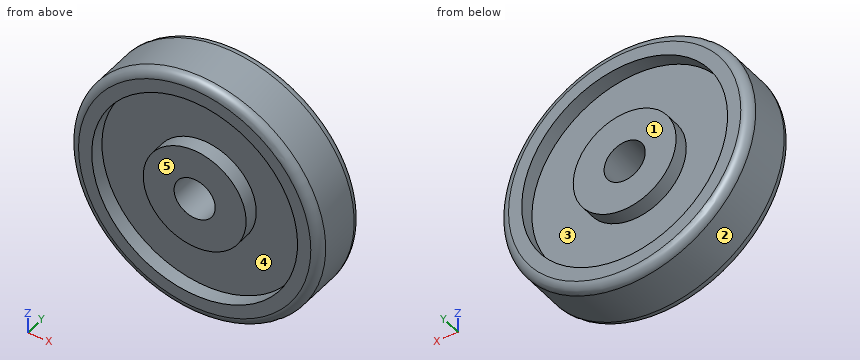
```python
from build123d import *

# Parameters (mm, degrees)
SKETCH_1_R          = 42.5
SKETCH_1_R_2        = 7
EXTRUDE_1_DEPTH     = 20
SKETCH_2_R          = 35
SKETCH_2_R_2        = 17.5
CUT_EXTRUDE_1_DEPTH = 5
CUT_EXTRUDE_START   = -5
SKETCH_3_R          = 35
SKETCH_3_R_2        = 17.5
CUT_EXTRUDE_2_DEPTH = 5
FILLET_1_R          = 3


with BuildPart() as part:
    # 草图1 → 凸台-拉伸1 (new body)
    with BuildSketch(Plane(origin=(0, 0, 0), x_dir=(1, 0, 0), z_dir=(0, 1, 0))):
        with Locations(Location((0, 0, 0), (0, 0, 270))):
            Circle(SKETCH_1_R)
        with Locations(Location((0, 0, 0), (0, 0, 270))):
            Circle(SKETCH_1_R_2, mode=Mode.SUBTRACT)
    extrude(amount=EXTRUDE_1_DEPTH)

    # 草图2 → 切除-拉伸1 (cut)
    with BuildSketch(Plane(origin=(0, 20, 0), x_dir=(1, 0, 0), z_dir=(0, 1, 0))):
        with Locations(Location((0, 0, 0), (0, 0, 270))):
            Circle(SKETCH_2_R)
        with Locations(Location((0, 0, 0), (0, 0, 270))):
            Circle(SKETCH_2_R_2, mode=Mode.SUBTRACT)
    extrude(amount=-CUT_EXTRUDE_1_DEPTH, mode=Mode.SUBTRACT)

    # 草图3 → 切除-拉伸2 (cut)
    with BuildSketch(Plane.XZ.offset(CUT_EXTRUDE_START)):
        with Locations(Location((0, 0, 0), (0, 0, 90))):
            Circle(SKETCH_3_R)
        with Locations(Location((0, 0, 0), (0, 0, 90))):
            Circle(SKETCH_3_R_2, mode=Mode.SUBTRACT)
    extrude(amount=CUT_EXTRUDE_2_DEPTH, mode=Mode.SUBTRACT)

    # 圆角1
    fillet_1_edges = [part.edges().sort_by_distance(p)[0] for p in [
        (0, 0, -42.5),
        (0, 20, -42.5),
    ]]
    fillet(fillet_1_edges, radius=FILLET_1_R)


solid = part.part
```
Could you check a few things on this model? Use its own coordinates, in mm. Face numbers are marked on the shaded views. A direction names the side the tool comes from. Give positions to 0.01 mm unless a question says otherwise; leave off trailing zeros. Order: outer loops, then holes, each group sorted by start corner. A loop starts at its lowest first (then second) coordinate and runs counter-clockwise, first axis right, second up.
Q1. If I drill on line 1 along X through (y, z) = (16.6, 0); line 2 along X through (y, z) = (4.75, 9.5); line 3 along Z through (x, y) = (-6, 1.25), over which ranges is the centre line in solid material (lowest first)?
Q2. Suppose I cut it at B-B, the plane z = 0. Write out the boundary of the cut face in (x, y), and give its area (3 significant figures).
Q3. For the marked faces 4 and 5, which set-ups out of +Z, -Z, +X, -X, +Y, -Y let a thin tool reach every point of the face, with its end or its side?
Q4. I'm going to push flat-ended pins straight in: P1, Ø3, axis at x = -24, z = -18.5, coming from the -Y side; P2, Ø12, axis at y = 15.5, z = 18.5, coming from the -X side; P3, Ø1.5, axis at x = 13.5, y = 16, coming from the +Z side. Where does each tip first touch, or does it pass through?
Q5. We'd pull the mould along X, two halves only. Please class the marked faces 1, 2 and 3: +X half, -X half, draft (parallel to the pull), parting line (faces both ways), or undercut.
Q6. Suppose I cut it at A-A, the plane x = 0. Write out the boundary of the cut face in (y, z), and give its area (3 significant figures).
Q7. Suppose I cut it at C-C, the plane y = 18. Write out the boundary of the cut face in (x, z), and give its area (3 significant figures).
Q8. Suppose I cut it at D-D, the plane y = 12. Write out the boundary of the cut face in (x, z), and give its area (3 significant figures).
Solution:
1. line 1: x = -42.5 to -35, -17.5 to -7, 7 to 17.5, 35 to 42.5
1. line 2: x = -41.42 to -33.69, -14.7 to 14.7, 33.69 to 41.42
1. line 3: z = -41.51 to -34.48, -16.44 to -3.61, 3.61 to 16.44, 34.48 to 41.51
2. outline: (-42.5, 3) arc R3 ccw to (-39.5, 0) - (-35, 0) - (-35, 5) - (-17.5, 5) - (-17.5, 0) - (-7, 0) - (-7, 20) - (-17.5, 20) - (-17.5, 15) - (-35, 15) - (-35, 20) - (-39.5, 20) arc R3 ccw to (-42.5, 17) - close; (7, 0) - (17.5, 0) - (17.5, 5) - (35, 5) - (35, 0) - (39.5, 0) arc R3 ccw to (42.5, 3) - (42.5, 17) arc R3 ccw to (39.5, 20) - (35, 20) - (35, 15) - (17.5, 15) - (17.5, 20) - (7, 20) - close
2. area: 1,060 mm2
3. face 4: -Y
3. face 5: +Z, -Z, +X, -X, -Y
4. P1: stops at y = 5
4. P2: stops at x = -40.62
4. P3: stops at z = 40.54
5. face 1: draft
5. face 2: parting line
5. face 3: undercut
6. outline: (0, -39.5) arc R3 ccw to (3, -42.5) - (17, -42.5) arc R3 ccw to (20, -39.5) - (20, -35) - (15, -35) - (15, -17.5) - (20, -17.5) - (20, -7) - (0, -7) - (0, -17.5) - (5, -17.5) - (5, -35) - (0, -35) - close; (0, 7) - (20, 7) - (20, 17.5) - (15, 17.5) - (15, 35) - (20, 35) - (20, 39.5) arc R3 ccw to (17, 42.5) - (3, 42.5) arc R3 ccw to (0, 39.5) - (0, 35) - (5, 35) - (5, 17.5) - (0, 17.5) - close
6. area: 1,060 mm2
7. outline: circle Ø84.66 at (0, 0); circle Ø35 at (0, 0); hole circle Ø70 at (0, 0); hole circle Ø14 at (0, 0)
7. area: 2,590 mm2
8. outline: circle Ø85 at (0, 0); hole circle Ø14 at (0, 0)
8. area: 5,520 mm2
